The listing builds one solid part. Answer for the finished solid, in the listing's coordinates (mm). A direction names the side the tool comes from. Give positions to 0.01 mm unless a question says otherwise; leave off trailing zeros. Order: outer loops, then holes, each group sorted by start corner. A loop starts at its lowest first (then second) coordinate and runs counter-clockwise, first axis right, second up. Notation, with made-up numbers: (61, 4) - (109, 4) arc R15 cw to (109, 30) - close; hole circle Ø8 at (26.25, 23.25). An arc over 180 degrees is marked (long way). Use a Markdown table: item, result. Add a question column.
1) Find section D-D, the plane x = 1.5. Determine the outline of the cut face in (y, z), plus the area to 3 significant figures.
2) For faces 1 (the face through (7, 25, -6)), 2 (the face through (3.6, 7, -3.6)), determine the directions among +Z, -Z, +X, -X, +Y, -Y from which every point of the face is accessible in a straight line to the end or side of a thin tool.
3) Flat-ended cylindrical pins translate along their axes: pin 1 (3 mm diameter, centred on x = 8.5, y = 10.5, fed in from -Z); pin 2 (4 mm diameter, centred on y = 19, z = -11, fed in from -X); pin 3 (1.5 mm diameter, centred on x = 9, y = 10, fed in from -Z). Find the tip coordinate at first contact, or state that the pin passes through.
4) Find section A-A, the plane z = -6.4. Determine the outline of the cut face in (x, y).
5) Find section B-B, the plane x = 6.6. Determine the outline of the cut face in (y, z), plus the area to 3 significant figures.
6) Find section C-C, the plane y = 23.5. Determine the outline of the cut face in (x, z).
7) Straight lines are drawn through the part: line 1 (Y direction, x = 5.75, z = -9.5); line 2 (Y direction, x = 9.25, z = -3.5); line 3 (X direction, y = 8.75, z = -8). For each, find the intervals that lie inside material, in ascending order.
from build123d import *

# Parameters (mm, degrees)
SKETCH1_W           = 13.2
SKETCH1_H           = 12.8
BOSS_EXTRUDE1_DEPTH = 7
SKETCH2_R           = 3.4
BOSS_EXTRUDE2_DEPTH = 18
CUT_EXTRUDE1_START  = -7.3
SKETCH3_R           = 3.4
SKETCH3_R_2         = 3
CUT_EXTRUDE1_DEPTH  = 7.3


with BuildPart() as part:
    # Sketch1 → Boss-Extrude1 (new body)
    with BuildSketch(Plane(origin=(0, 0, 0), x_dir=(1, 0, 0), z_dir=(0, 1, 0))):
        with Locations((6.6, 6.4)):
            Rectangle(SKETCH1_W, SKETCH1_H)
    extrude(amount=BOSS_EXTRUDE1_DEPTH)

    # Sketch2 → Boss-Extrude2 (add)
    with BuildSketch(Plane(origin=(0, 7, 0), x_dir=(1, 0, 0), z_dir=(0, 1, 0))):
        with Locations(Location((6.6, 6.4, 0), (0, 0, 90))):
            Circle(SKETCH2_R)
    extrude(amount=BOSS_EXTRUDE2_DEPTH)

    # Sketch3 → Cut-Extrude1 (cut)
    with BuildSketch(Plane(origin=(0, 25, 0), x_dir=(1, 0, 0), z_dir=(0, 1, 0)).offset(CUT_EXTRUDE1_START)):
        with Locations(Location((6.6, 6.4, 0), (0, 0, 90))):
            Circle(SKETCH3_R)
        with Locations(Location((6.6, 6.4, 0), (0, 0, 270))):
            Circle(SKETCH3_R_2, mode=Mode.SUBTRACT)
    extrude(amount=CUT_EXTRUDE1_DEPTH, mode=Mode.SUBTRACT)

    # Sketch7 → Cut-Revolve2 (revolve, cut)
    with BuildSketch(Plane.XY.offset(-6.4), mode=Mode.PRIVATE) as cut_revolve2_sk:
        Polygon((8.6, 25), (9.6, 24), (9.6, 25), align=None)
    revolve(cut_revolve2_sk.sketch.rotate(Axis((6.6, 25, -6.4), (0, 1, 0)), 270), axis=Axis((6.6, 25, -6.4), (0, 1, 0)), mode=Mode.SUBTRACT)


solid = part.part
The answers:
| question | item | result |
|---|---|---|
| 1 | outline | (0, -12.8) - (7, -12.8) - (7, 0) - (0, 0) - close |
| 1 | area | 89.6 mm2 |
| 2 | face 1 | +Z, -Z, +X, -X, +Y |
| 2 | face 2 | +Y |
| 3 | pin 1 | z = -9.78 |
| 3 | pin 2 | x = 5.1 |
| 3 | pin 3 | z = -9.37 |
| 4 | outline | (0, 0) - (13.2, 0) - (13.2, 7) - (10, 7) - (10, 17.7) - (9.6, 17.7) - (9.6, 24) - (8.6, 25) - (4.6, 25) - (3.6, 24) - (3.6, 17.7) - (3.2, 17.7) - (3.2, 7) - (0, 7) - close |
| 5 | outline | (0, -12.8) - (7, -12.8) - (7, -9.8) - (17.7, -9.8) - (17.7, -9.4) - (24, -9.4) - (25, -8.4) - (25, -4.4) - (24, -3.4) - (17.7, -3.4) - (17.7, -3) - (7, -3) - (7, 0) - (0, 0) - close |
| 5 | area | 205 mm2 |
| 6 | outline | circle Ø6 at (6.6, -6.4) |
| 7 | line 1 | 0 to 17.7 |
| 7 | line 2 | 0 to 7 |
| 7 | line 3 | 3.6 to 9.6 |
